Source: CAD feature listing. Evaluate the final solid. Frame: model axes, mm. A direction names the side the tool comes from. Round coordinates to 2 decimals unless told otherwise and drop trailing zeros. Write each loop counter-clockwise with the first axis right and the second up, starting at its lowest first coordinate (ties: lowest second). Pieces come first, ordered by that corner, then holes. Notation, with made-up numbers: (77.25, -21.5) - (117.25, -21.5) arc R37 ccw to (117.25, 16.5) - close; hole circle Ø11 at (6, 67). An arc over 180 degrees is marked (long way). Write item = value, one per line. Start each with the question number.
```python
from build123d import *

# Parameters (mm, degrees)
EXTRUDE_1_DEPTH                  = 10
FILLET_1_R                       = 2
PATTERN_CIRCULAR_2_COUNT         = 3
FILLET_1_OF_PATTERN_CIRCULAR_2_R = 2
CUT_EXTRUDE_START                = -15
SKETCH_3_R                       = 51
CUT_EXTRUDE_1_DEPTH              = 15
SKETCH_4_R                       = 62.618720145
SKETCH_4_R_2                     = 57
CUT_EXTRUDE_2_DEPTH              = 15
CHAMFER_1_SIZE                   = 2
FILLET_2_R                       = 5
SKETCH_5_R                       = 42.5
EXTRUDE_2_DEPTH                  = 3


with BuildPart() as part:
    # Sketch 1 → Revolve 1 (revolve)
    with BuildSketch(Plane(origin=(0, 0, 0), x_dir=(1, 0, 0), z_dir=(0, 1, 0))):
        Polygon((0, 0), (-54, 0), (-54, 145), (-51, 145), (-51, 3), (0, 3), align=None)
    revolve(axis=Axis((0, 0, -3), (0, 0, 1)))

    # Sketch 2 → Extrude 1 (add)
    with BuildSketch(Plane(origin=(57, 0, 0), x_dir=(0, 0, -1), z_dir=(1, 0, 0))):
        Polygon((145, 14), (145, -14), (140, -14), (138.5, 11), (134, 11), (134, 14), align=None)
    extrude_1 = extrude(amount=-EXTRUDE_1_DEPTH)

    # Fillet 1
    fillet_1_edges = [part.edges().sort_by_distance(p)[0] for p in [
        (54.576809621, -14, -140),
    ]]
    fillet(fillet_1_edges, radius=FILLET_1_R)

    # Pattern Circular 2: Extrude 1 ×3 about axis
    pattern_circular_2_axis = Axis((0, 0, 0), (0, 0, 1))
    for i in range(1, PATTERN_CIRCULAR_2_COUNT):
        add(extrude_1.rotate(pattern_circular_2_axis, i * 360 / PATTERN_CIRCULAR_2_COUNT))

    # Fillet 1 of Pattern Circular 2
    fillet_1_of_pattern_circular_2_edges = [part.edges().sort_by_distance(p)[0] for p in [
        (-15.164049157, 54.264903589, -140),
        (-39.412760463, -40.264903589, -140),
    ]]
    fillet(fillet_1_of_pattern_circular_2_edges, radius=FILLET_1_OF_PATTERN_CIRCULAR_2_R)

    # Sketch 3 → Cut-Extrude 1 (cut)
    with BuildSketch(Plane(origin=(0, 0, -145), x_dir=(-1, 0, 0), z_dir=(0, 0, -1)).offset(CUT_EXTRUDE_START)):
        Circle(SKETCH_3_R)
    extrude(amount=CUT_EXTRUDE_1_DEPTH, mode=Mode.SUBTRACT)

    # Sketch 4 → Cut-Extrude 2 (cut)
    with BuildSketch(Plane(origin=(0, 0, -145), x_dir=(-1, 0, 0), z_dir=(0, 0, -1))):
        Circle(SKETCH_4_R)
        Circle(SKETCH_4_R_2, mode=Mode.SUBTRACT)
    extrude(amount=-CUT_EXTRUDE_2_DEPTH, mode=Mode.SUBTRACT)

    # Chamfer 1
    chamfer_1_edges = [part.edges().sort_by_distance(p)[0] for p in [
        (54, 0, 0),
    ]]
    chamfer(chamfer_1_edges, length=CHAMFER_1_SIZE)

    # Fillet 2
    fillet_2_edges = [part.edges().sort_by_distance(p)[0] for p in [
        (51, 0, -3),
    ]]
    fillet(fillet_2_edges, radius=FILLET_2_R)

    # Sketch 5 → Extrude 2 (add)
    with BuildSketch(Plane.XY):
        Circle(SKETCH_5_R)
    extrude(amount=EXTRUDE_2_DEPTH)


solid = part.part
```
(1) Contact query for flat-ended pins moving along their axis: P1, Ø4, axis at x = -16.5, y = -53, coming from the +Z side; P2, Ø1, axis at x = -28, z = -125, coming from the -Y side; P3, Ø3.5, axis at x = 54, z = -143.5, coming from the -Y side. Output: stop coordinate, or through.
(2) Section B-B (x = 0). Return the cut outline in (y, z).
(3) Pull-direction query (Y, two-part tool) for faces 1 (the flat face through (1, -1, -3)), 2 (the flat face through (-38, 41, -134)), 3 (the cylindrical face through (-33.727, -25.861, 1.479)), 4 (the cylindrical face through (11.056, 49.787, -75.541)); classes: +Y half, -Y half, draft (parallel to the pull), parting line (faces both ways), or undercut.
(4) Section A-A (y = 0). Return the cut outline in (x, z).
(5) Section C-C (z = -63.5). Return the cut outline in (x, y), plus the area to 3 significant figures.
(6) Ray query, L1, parallel to X at y = 0, z = -114; L2, parallel to Z at x = 17, y = -10; L3, parallel to Z at x = 25.5, y = 36. Return the intervals inside material, ascending. Write a range as from..to.
(7) Reachability of faces 5 (the cylindrical face through (11.706, 52.716, -74.501)), 6 (the cylindrical face through (57, 0, -142)), 7 (the flat face through (-16, -53, -134)) from +Z, -Z, +X, -X, +Y, -Y: full face, straight path, thin tool, end or side. Return the list, or none.
Solution:
q1.P1 = -1.51
q1.P2 = -46.47
q1.P3 = -14
q2.outline = (-54, -145) - (-51, -145) - (-51, -8) arc R5 cw to (-46, -3) - (46, -3) arc R5 cw to (51, -8) - (51, -145) - (54, -145) - (54, -2) - (52, 0) - (42.5, 0) - (42.5, 3) - (-42.5, 3) - (-42.5, 0) - (-52, 0) - (-54, -2) - close
q3.face_1 = undercut
q3.face_2 = draft
q3.face_3 = parting line
q3.face_4 = undercut
q4.outline = (-54, -145) - (-51, -145) - (-51, -8) arc R5 cw to (-46, -3) - (46, -3) arc R5 cw to (51, -8) - (51, -145) - (57, -145) - (57, -139.16) - (54, -139.16) - (54, -2) - (52, 0) - (42.5, 0) - (42.5, 3) - (-42.5, 3) - (-42.5, 0) - (-52, 0) - (-54, -2) - close
q5.outline = circle Ø108 at (0, 0); hole circle Ø102 at (0, 0)
q5.area = 990 mm^2
q6.L1 = -54..-51, 51..54
q6.L2 = -3..3
q6.L3 = -3..0
q7.face_5 = +Z
q7.face_6 = +Z, -Z, +X
q7.face_7 = +Z, -X, -Y
